Geometry: final body of the model. Coordinates: model frame, mm. Face numbers are marked on the shaded views. A direction names the side the tool comes from. Round coordinates to 2 decimals unless told otherwise and drop trailing zeros. Write each loop counter-clockwise with the first axis right and the second up, starting at its lowest first coordinate (ties: lowest second). Pieces come first, ordered by that corner, then holes. Notation, with made-up numbers: M 24,-4.75 L 52,-4.75 A22 cw 52,26.25 Z; hole C 26.25,13.5 d2. An arc over 180 degrees is marked long. Put each result on its own line as item: value. Start each with the question number.
```python
from build123d import *

# Parameters (mm, degrees)
F0_W      = 127
F0_H      = 127
F2_DEPTH  = 127
F6_R      = 10.16
F7_DEPTH  = 6.35
F8_R      = 10.16
F9_DEPTH  = 6.35
F10_R     = 10.16
F11_DEPTH = 6.35
F12_R     = 10.16
F13_DEPTH = 6.35
F14_R     = 10.16
F15_DEPTH = 6.35
F16_R     = 10.16
F17_DEPTH = 6.35


with BuildPart() as f2:
    # F0 (on Top) → F2 (new body)
    with BuildSketch(Plane.XY):
        Rectangle(F0_W, F0_H)
    extrude(amount=F2_DEPTH)


with BuildPart() as f4:
    # F3 (on offset) → F4 (revolve)
    with BuildSketch(Plane.XY.offset(63.5)):
        with BuildLine():
            Line((0, -90.937567), (0, 90.937567))
            ThreePointArc((0, 90.937567), (-90.937567, 0), (0, -90.937567))
        make_face()
    revolve(axis=Axis((0, 0, 63.5), (0, -1, 0)))

    # F5: intersect F2
    add(f2.part, mode=Mode.INTERSECT)

    # F6 (on face) → F7 (cut)
    with BuildSketch(Plane(origin=(0, 63.5, 0), x_dir=(-1, 0, 0), z_dir=(0, 1, 0))):
        with Locations((0, 63.5)):
            Circle(F6_R)
    extrude(amount=-F7_DEPTH, mode=Mode.SUBTRACT)

    # F8 (on face) → F9 (cut)
    with BuildSketch(Plane.XZ.offset(63.5)):
        with Locations((31.75, 95.25)):
            Circle(F8_R)
        with Locations((31.75, 63.5)):
            Circle(F8_R)
        with Locations((31.75, 31.75)):
            Circle(F8_R)
        with Locations((-31.75, 31.75)):
            Circle(F8_R)
        with Locations((-31.75, 63.5)):
            Circle(F8_R)
        with Locations((-31.640418, 94.16756)):
            Circle(F8_R)
    extrude(amount=-F9_DEPTH, mode=Mode.SUBTRACT)

    # F10 (on face) → F11 (cut)
    with BuildSketch(Plane.XY.offset(127)):
        Circle(F10_R)
        with Locations((31.75, 31.75)):
            Circle(F10_R)
        with Locations((31.75, -31.75)):
            Circle(F10_R)
        with Locations((-31.75, -31.75)):
            Circle(F10_R)
        with Locations((-31.75, 31.75)):
            Circle(F10_R)
    extrude(amount=-F11_DEPTH, mode=Mode.SUBTRACT)

    # F12 (on face) → F13 (cut)
    with BuildSketch(Plane(origin=(0, 0, 0), x_dir=(1, 0, 0), z_dir=(0, 0, -1))):
        with Locations((31.75, 31.75)):
            Circle(F12_R)
        with Locations((-31.75, -31.75)):
            Circle(F12_R)
    extrude(amount=-F13_DEPTH, mode=Mode.SUBTRACT)

    # F14 (on face) → F15 (cut)
    with BuildSketch(Plane.YZ.offset(63.5)):
        with Locations((0, 63.5)):
            Circle(F14_R)
        with BuildLine():
            ThreePointArc((31.75, 85.09), (38.934205, 88.065795), (41.91, 95.25))
            ThreePointArc((41.91, 95.25), (24.565795, 102.434205), (31.75, 85.09))
        make_face()
        with BuildLine():
            ThreePointArc((-31.75, 41.91), (-38.934205, 24.565795), (-21.59, 31.75))
            ThreePointArc((-21.59, 31.75), (-24.565795, 38.934205), (-31.75, 41.91))
        make_face()
    extrude(amount=-F15_DEPTH, mode=Mode.SUBTRACT)

    # F16 (on face) → F17 (cut)
    with BuildSketch(Plane(origin=(-63.5, 0, 0), x_dir=(0, -1, 0), z_dir=(-1, 0, 0))):
        with Locations((-31.75, 95.25)):
            Circle(F16_R)
        with Locations((-31.75, 31.75)):
            Circle(F16_R)
        with Locations((31.75, 31.75)):
            Circle(F16_R)
        with Locations((31.75, 95.25)):
            Circle(F16_R)
    extrude(amount=-F17_DEPTH, mode=Mode.SUBTRACT)


solid = f4.part
```
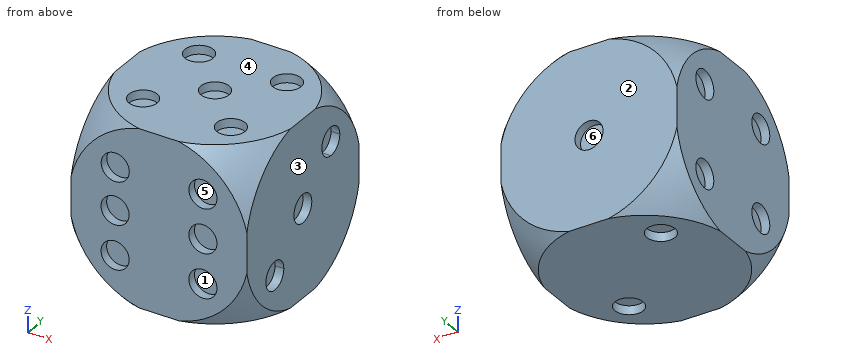
1) Access query for the marked faces 4, 5 and 6. Directions: +Z, -Z, +X, -X, +Y, -Y. A direction counts if a zero-diameter tool reaches every point of the face in a straight line with its end or side. Return the directions, or none.
2) Draft query along X for the marked faces 1, 2 and 3. Return one class per face: +X half, -X half, draft (parallel to the pull), parting line (faces both ways), or undercut.
3) Section B-B, the plane z = 12. Output: boundary loops of the cut face in (x, y), and give its area (3 significant figures).
4) Section C-C, the plane y = -52. Output: boundary loops of the cut face in (x, z).
5) First-contact query: pin 1 (16.5 mm diameter, centred on y = -34.5, z = 32, fed in from -X); pin 2 (2 mm diameter, centred on x = -30, z = 69, fed in from -Y); pin 3 (18.5 mm diameter, centred on x = 31.75, y = -31.75, fed in from -Z); pin 4 (18.5 mm diameter, centred on x = -31.75, y = 31.75, fed in from +Z). Flat tips, straight axial feed; report the tip coordinate or a pass-through.
6) Ray query, probe 1 along Y at (x, z) = (-60, 31); probe 2 along Y at (x, z) = (-61, 95); probe 3 along X at (y, z) = (31, 122). Return the intervals inside material, ascending.
7) Section A-A, the plane x = 0. Output: boundary loops of the cut face in (y, z), and give its area (3 significant figures).
Solved:
1. face 4: +Z, +X, -X, +Y, -Y
1. face 5: -Y
1. face 6: +Y
2. face 1: undercut
2. face 2: draft
2. face 3: +X half
3. outline: M -63.5,-39.81 A74.95 ccw -39.81,-63.5 L 39.81,-63.5 A74.95 ccw 63.5,-39.81 L 63.5,39.81 A74.95 ccw 39.81,63.5 L -39.81,63.5 A74.95 ccw -63.5,39.81 Z
3. area: 15,200 mm2
4. outline: M -63.5,24.34 A74.6 ccw -39.16,0 L 39.16,0 A74.6 ccw 63.5,24.34 L 63.5,102.66 A74.6 ccw 39.16,127 L -39.16,127 A74.6 ccw -63.5,102.66 Z
5. pin 1: stops at x = -63.5
5. pin 2: stops at y = -57.15
5. pin 3: stops at z = 6.35
5. pin 4: stops at z = 120.65
6. probe 1: y = -60.11 to -41.88, -21.62 to 21.62, 41.88 to 60.11
6. probe 2: y = -59.64 to -41.91, -21.59 to 21.59, 41.91 to 59.64
6. probe 3: x = -62.34 to -41.88, -21.62 to 21.62, 41.88 to 62.34
7. outline: M -63.5,0 L 63.5,0 L 63.5,53.34 L 57.15,53.34 L 57.15,73.66 L 63.5,73.66 L 63.5,127 L 10.16,127 L 10.16,120.65 L -10.16,120.65 L -10.16,127 L -63.5,127 Z
7. area: 15,900 mm2
